Can you work these out from the model? Positions are in its coordinate system, mm. Coordinates: 2 decimals unless noted, no trailing zeros. Order: outer loops, then holes, each group sorted by start corner. A loop starts at its lowest first (then second) coordinate and runs counter-clockwise, first axis right, second up. Notation, with made-up numbers: (-4.5, 71) - (7.5, 71) arc R7 ccw to (7.5, 77) - close; hole circle Ø8 at (6, -21.75). An arc over 180 degrees is marked (long way). Use a Markdown table: item, result. Add a question column.
(1) I want a section at A-A (x = 66.5). List the corners of the cut face in (y, z) for me.
(2) If I drill on L1, parallel to Y at x = -51, z = -5; L2, parallel to Z at x = 49.5, y = 12.25; L3, parallel to Y at x = -41, z = -35, over which ranges is the centre line in solid material (lowest first)? Write a range as [from, to].
(3) For pin 1 Ø1.5 at (x, z) = (58.5, -31.5) entering from -Y; pin 2 Ø0.9 at (x, y) = (49.5, 11.5) entering from +Z; pin 3 Ø7 at (x, z) = (-82.05, -12.57) entering from +Y; pin 4 Ø3 at (x, z) = (-9, 12.5) entering from +Y, each with a flat end and sliding along its axis, tell me the tip position at first contact or that it passes through.
(4) I want a section at B-B (x = -49). List the corners of the cut face in (y, z) for me.
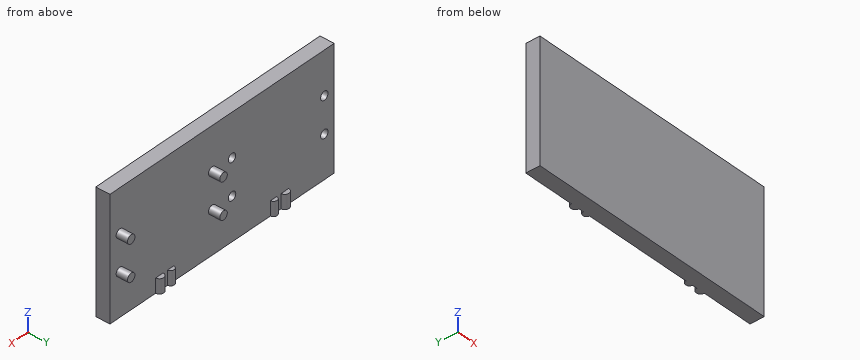
```python
from build123d import *

# Parameters (mm, degrees)
SCHIZZO1_W                   = 180
SCHIZZO1_H                   = 85
ESTRUSIONE_ESTRUSIONE1_DEPTH = 10
SCHIZZO5_R                   = 3
ESTRUSIONE_ESTRUSIONE3_DEPTH = 8
SCHIZZO5_3_R                 = 3
TAGLIO_ESTRUSIONE1_DEPTH     = 8
ESTRUSIONE_ESTRUSIONE4_DEPTH = 10


with BuildPart() as part:
    # Schizzo1 → Estrusione-Estrusione1 (new body)
    with BuildSketch(Plane(origin=(0, 0, 0), x_dir=(1, 0, 0), z_dir=(0, 1, 0))):
        Rectangle(SCHIZZO1_W, SCHIZZO1_H)
    extrude(amount=ESTRUSIONE_ESTRUSIONE1_DEPTH)

    # Schizzo5 → Estrusione-Estrusione3 (add)
    with BuildSketch(Plane(origin=(0, 10, 0), x_dir=(1, 0, 0), z_dir=(0, 1, 0))):
        with Locations(Location((82.045349051, -12.571464774, 0), (0, 0, 270))):
            Circle(SCHIZZO5_R)
        with Locations(Location((82.045349051, 12.571464774, 0), (0, 0, 90))):
            Circle(SCHIZZO5_R)
        with Locations(Location((7.954650949, -12.571464774, 0), (0, 0, 90))):
            Circle(SCHIZZO5_R)
        with Locations(Location((7.954650949, 12.571464774, 0), (0, 0, 270))):
            Circle(SCHIZZO5_R)
    extrude(amount=ESTRUSIONE_ESTRUSIONE3_DEPTH)

    # Schizzo5_3 → Taglio-Estrusione1 (cut)
    with BuildSketch(Plane(origin=(0, 10, 0), x_dir=(1, 0, 0), z_dir=(0, 1, 0))):
        with Locations(Location((-82.045349051, 12.571464774, 0), (0, 0, 270))):
            Circle(SCHIZZO5_3_R)
        with Locations(Location((-82.045349051, -12.571464774, 0), (0, 0, 90))):
            Circle(SCHIZZO5_3_R)
        with Locations(Location((-7.954650949, -12.571464774, 0), (0, 0, 270))):
            Circle(SCHIZZO5_3_R)
        with Locations(Location((-7.954650949, 12.571464774, 0), (0, 0, 90))):
            Circle(SCHIZZO5_3_R)
    extrude(amount=-TAGLIO_ESTRUSIONE1_DEPTH, mode=Mode.SUBTRACT)

    # Schizzo6 → Estrusione-Estrusione4 (add)
    with BuildSketch(Plane(origin=(0, 0, -42.5), x_dir=(-1, 0, 0), z_dir=(0, 0, -1))):
        with BuildLine():
            Line((-53.319235265, 10), (-47.319235265, 10))
            ThreePointArc((-47.319235265, 10), (-50.319235265, 13), (-53.319235265, 10))
        make_face()
        with BuildLine():
            Line((-43.794702793, 10), (-38.794702793, 10))
            ThreePointArc((-38.794702793, 10), (-41.294702793, 12.5), (-43.794702793, 10))
        make_face()
        with BuildLine():
            Line((43.794702793, 10), (38.794702793, 10))
            ThreePointArc((38.794702793, 10), (41.294702793, 12.5), (43.794702793, 10))
        make_face()
        with BuildLine():
            Line((53.319235265, 10), (47.319235265, 10))
            ThreePointArc((47.319235265, 10), (50.319235265, 13), (53.319235265, 10))
        make_face()
    extrude(amount=-ESTRUSIONE_ESTRUSIONE4_DEPTH)


solid = part.part
```
Answers follow:
| question | item | result |
|---|---|---|
| 1 | outline | (0, -42.5) - (10, -42.5) - (10, 42.5) - (0, 42.5) - close |
| 2 | L1 | y = [0, 10] |
| 2 | L2 | z = [-42.5, -32.5] |
| 2 | L3 | y = [0, 12.48] |
| 3 | pin 1 | stops at y = 0 |
| 3 | pin 2 | stops at z = -32.5 |
| 3 | pin 3 | stops at y = 10 |
| 3 | pin 4 | stops at y = 2 |
| 4 | outline | (0, -42.5) - (12.69, -42.5) - (12.69, -32.5) - (10, -32.5) - (10, 42.5) - (0, 42.5) - close |
